Part model, mm, in its own coordinate system. Face numbers are marked on the shaded views. A direction names the side the tool comes from. Coordinates: 2 decimals unless noted, no trailing zeros. Loops run counter-clockwise (first coordinate to the right, second up) from the corner with the lowest first, then second, coordinate; pieces in that order, holes last. Notation, with made-up numbers: (-19.5, 87.25) - (7.5, 87.25) arc R23 cw to (7.5, 122.25) - close; hole circle Ø2 at (78, -1.75). An arc over 180 degrees is marked (long way). Answer as CSV lines item,"result".
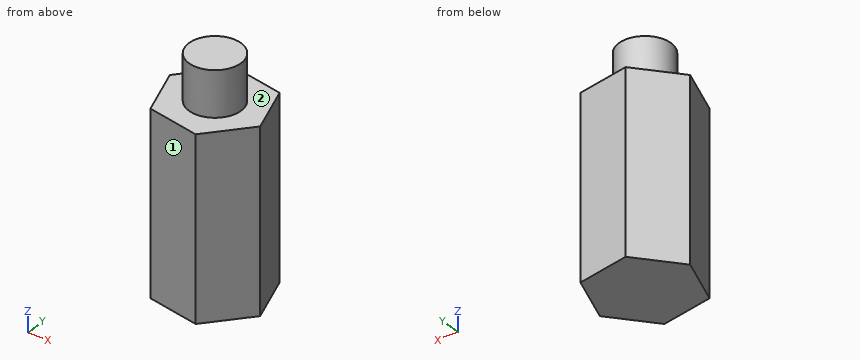
from build123d import *

# Parameters (mm, degrees)
F0_R     = 26.8270894081
F1_DEPTH = 55.372
F2_R     = 20.1512437213
F3_DEPTH = 90.424
F4_DEPTH = 84.328


with BuildPart() as f1:
    # F0 (on Top) → F1 (new body)
    with BuildSketch(Plane.XY):
        Polygon((-13.5254997487, 39.0910579561), (-40.6165991252, 7.8321025968), (-27.0910993765, -31.2589553593), (13.5254997487, -39.0910579561), (40.6165991252, -7.8321025968), (27.0910993765, 31.2589553593), align=None)
        Circle(F0_R, mode=Mode.SUBTRACT)
        Circle(F0_R)
    extrude(amount=F1_DEPTH)

    # F2 (on Top) → F3 (join)
    with BuildSketch(Plane.XY):
        Circle(F2_R)
    extrude(amount=F3_DEPTH)

    # F4 (add): a face of the model
    f4_faces = [f1.faces().sort_by_distance(p)[0] for p in [
        (0, 0, 0),
    ]]
    extrude(f4_faces, amount=F4_DEPTH)


solid = f1.part
Q1. Flat gauge pins, fed straight in: pin 1 (8 mm diameter, centred on x = -23, y = 21, fed in from +Z); pin 2 (5 mm diameter, centred on x = -23.5, z = -57, fed in from -Y); pin 3 (10 mm diameter, centred on x = -11.5, z = -63, fed in from +Y); pin 4 (6 mm diameter, centred on x = -1, z = 56.5, fed in from -Y). Where does each tip first touch, or does it go through?
Results:
pin 1,"stops at z = 55.37"
pin 2,"stops at y = -32.43"
pin 3,"stops at y = 39.09"
pin 4,"stops at y = -36.83"
Q2. Wall check: L1, parallel to Z at x = -9, y = -25.5; L2, parallel to X at y = -10, z = 77; L3, parallel to Y at x = 11.5, z = -45. Give the ranges that are in metal, low to high.
Results:
L1,"z = -84.33 to 55.37"
L2,"x = -17.49 to 17.49"
L3,"y = -38.7 to 34.27"
Q3. Saw through at B-B (y = 4.5). Give the cut face in (x, z), then the cut area to 3 significant figures.
Results:
outline,"(-39.46, -84.33) - (36.35, -84.33) - (36.35, 55.37) - (19.64, 55.37) - (19.64, 90.42) - (-19.64, 90.42) - (-19.64, 55.37) - (-39.46, 55.37) - close"
area,"12,000 mm^2"
Q4. Which spindle directions (+Z, -Z, +X, -X, +Y, -Y) get a long thin tool onto all of the face, cutting with end or side? Do the marked faces 1 and 2. Say none if no direction does.
Results:
face 1,"+Z, -Z, -X, -Y"
face 2,"+Z"
Q5. Saw through at D-D (x = 35.5). Give the cut face in (y, z).
Results:
outline,"(-13.74, -84.33) - (6.96, -84.33) - (6.96, 55.37) - (-13.74, 55.37) - close"
Q6. Saw through at C-C (x = 0). Give the cut face in (y, z).
Results:
outline,"(-36.48, -84.33) - (36.48, -84.33) - (36.48, 55.37) - (20.15, 55.37) - (20.15, 90.42) - (-20.15, 90.42) - (-20.15, 55.37) - (-36.48, 55.37) - close"
Q7. Saw through at A-A (z = -21). Give the cut face in (x, y).
Results:
outline,"(-40.62, 7.83) - (-27.09, -31.26) - (13.53, -39.09) - (40.62, -7.83) - (27.09, 31.26) - (-13.53, 39.09) - close"
